Can you work these out from the model? Positions are in its coordinate system, mm. Face numbers are marked on the shaded views. A direction names the side the tool comes from. Give positions to 0.01 mm unless a question says otherwise; leave off trailing zeros. Loops run counter-clockwise (first coordinate to the right, second up) from the corner with the lowest first, then second, coordinate; pieces in that order, holes last. Notation, with made-up numbers: (89, 24.25) -> (117, 24.25) arc R29 ccw to (117, 48.25) -> close; hole circle Ø6 at (16.25, 68.5). An arc over 180 degrees is marked (long way). Return JSON: item names as keys, results as strings. Group by question number.
Q1. Thinking about a two-plate mould opening in Y: for the marked faces 4, 5 and 6, which applies, pulls with the +Y half, pulls with the -Y half, needs draft (parallel to the pull), parting line crosses it, or undercut?
Q2. Suppose I cut it at A-A, the plane z = 56. Please give me the cut outline in (x, y).
Q3. Will these pins go through, and if not, where does the flat tip stop? pin 1 (3 mm diameter, centred on y = 9, z = 52.5, fed in from -X); pin 2 (4.5 mm diameter, centred on x = -5, y = 13.5, fed in from +Z); pin 3 (10.5 mm diameter, centred on x = -0.5, y = 9, fed in from +Z).
Q4. I need wall thicknesses on line 1 along Z through (x, y) = (-5, 9); line 2 along Z through (x, y) = (4, -11.5); line 3 along X through (y, z) = (-10.5, 11). Which ranges of each line are inside material? Lowest first, please. Write a range as [from, to].
Q5. Suppose I cut it at B-B, the plane z = -11. Please give me the cut outline in (x, y), and give its area (3 significant figures).
Q6. Which directions (+Z, -Z, +X, -X, +Y, -Y) give clear straight access to the entire face, cutting with the end or side of a thin tool? Please do the marked faces 1, 2 and 3.
```python
from build123d import *

# Parameters (mm, degrees)
F2_W            = 4.3805325404
F2_H            = 13.738937676
F3_ANGLE        = 30
F3_COPIES_COUNT = 6
F5_ANGLE        = 30
F5_COPIES_COUNT = 4


# Not quite as in the source:
# - a pattern or mirror of a feature is missing from the dataset's text; its kind, count and spacing are read off the source's solid


with BuildPart() as f1:
    # F0 (on Front) → F1 (revolve)
    with BuildSketch(Plane.XZ):
        Polygon((0, 72.776556015), (0, 67.1017691493), (6.2909605913, 67.1017691493), align=None)
        Polygon((0, 67.1017691493), (0, 51.4894537628), (7.8760384344, 51.4894537628), (17.8207978606, 67.1017691493), (6.2909605913, 67.1017691493), align=None)
        with BuildLine():
            Line((0, 51.4894537628), (0, -17.9203543812))
            Line((0, -17.9203543812), (25.1880511642, -17.9203543812))
            Line((25.1880511642, -17.9203543812), (23.1969021261, -13.3407087997))
            ThreePointArc((23.1969021261, -13.3407087997), (19.2033042996, -12.428933787), (17.024340108, -8.9601771906))
            Line((17.024340108, -8.9601771906), (15.7520768689, -1.4651455679))
            Line((15.7520768689, -1.4651455679), (18.0199127644, 10.7748573646))
            Line((18.0199127644, 10.7748573646), (15.7520768689, 18.9159307629))
            ThreePointArc((15.7520768689, 18.9159307629), (17.3860110627, 23.4955772758), (15.7520768689, 28.0752237886))
            Line((15.7520768689, 28.0752237886), (12.3262992129, 38.1487458944))
            Line((12.3262992129, 38.1487458944), (15.7520768689, 51.4894537628))
            Line((15.7520768689, 51.4894537628), (7.8760384344, 51.4894537628))
            Line((7.8760384344, 51.4894537628), (0, 51.4894537628))
        make_face()
    revolve(axis=Axis((0, 0, 27.4281008169), (0, 0, -1)))

    # F2 (on Front) → F3 (revolve)
    with BuildSketch(Plane.XZ):
        with Locations((13.8384955935, 37.1349565685)):
            Rectangle(F2_W, F2_H)
    f3 = revolve(axis=Axis((0, 0, 27.4281008169), (0, 0, -1)), revolution_arc=F3_ANGLE)

    # F3_copies: F3 ×6 about axis
    f3_copies_axis = Axis((0, 0, 0), (0, 0, 1))
    for i in range(1, F3_COPIES_COUNT):
        add(f3.rotate(f3_copies_axis, i * 360 / F3_COPIES_COUNT))

    # F4 (on Front) → F5 (revolve)
    with BuildSketch(Plane.XZ):
        Polygon((12.8429187462, 49.7787632048), (8.263274096, 58.5398264229), (6.6703548655, 49.7787632048), align=None)
    f5 = revolve(axis=Axis((0, 0, 27.4281008169), (0, 0, -1)), revolution_arc=F5_ANGLE)

    # F5_copies: F5 ×4 about axis
    f5_copies_axis = Axis((0, 0, 0), (0, 0, 1))
    for i in range(1, F5_COPIES_COUNT):
        add(f5.rotate(f5_copies_axis, i * 360 / F5_COPIES_COUNT))


solid = f1.part
```
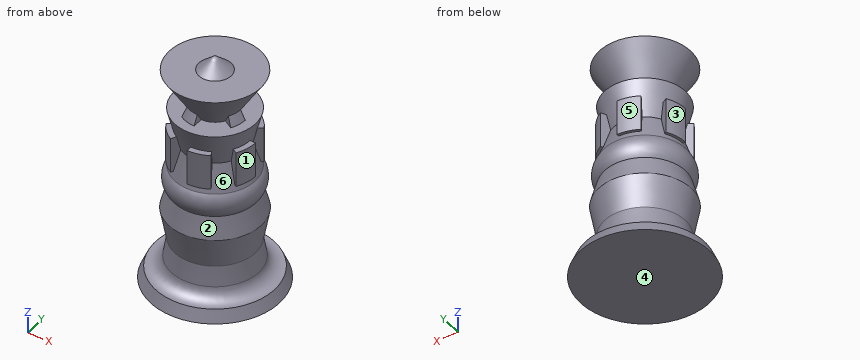
Ans:
{
 "1": {"face 4": "needs draft", "face 5": "pulls with the +Y half", "face 6": "undercut"},
 "2": {"outline": "circle Ø21.5 at (0, 0)"},
 "3": {"pin 1": "stops at x = -13.63", "pin 2": "stops at z = 67.1", "pin 3": "stops at z = 69.38"},
 "4": {"line 1": "z = [-17.92, 51.49], [55.29, 67.1]", "line 2": "z = [-17.92, 51.49], [58.24, 67.1]", "line 3": "x = [-14.57, 14.57]"},
 "5": {"outline": "circle Ø35.65 at (0, 0)", "area": "998 mm^2"},
 "6": {"face 1": "+X, -Y", "face 2": "none", "face 3": "-X, +Y"}
}
